from build123d import *

# Parameters (mm, degrees)
BOX013_W     = 26
BOX013_H     = 26
BOX013_DEPTH = 3
BOX014_W     = 5
BOX014_H     = 5
BOX014_DEPTH = 9
BOX012_W     = 30
BOX012_H     = 30
BOX012_DEPTH = 2
BOX015_W     = 5
BOX015_H     = 5
BOX015_DEPTH = 9
FILLET001_R  = 2
FILLET002_R  = 2


with BuildPart() as obj1:
    # Box013 → Box013 (new body)
    with BuildSketch(Plane(origin=(-13, -13, -10), x_dir=(1, 0, 0), z_dir=(0, 0, 1))):
        with Locations((13, 13)):
            Rectangle(BOX013_W, BOX013_H)
    extrude(amount=BOX013_DEPTH)


with BuildPart() as obj2:
    # Box014 → Box014 (new body)
    with BuildSketch(Plane(origin=(-13, 8, -7), x_dir=(1, 0, 0), z_dir=(0, 0, 1))):
        with Locations((2.5, 2.5)):
            Rectangle(BOX014_W, BOX014_H)
    extrude(amount=BOX014_DEPTH)


with BuildPart() as obj3:
    # Box012 → Box012 (new body)
    with BuildSketch(Plane(origin=(-15, -15, -12), x_dir=(1, 0, 0), z_dir=(0, 0, 1))):
        with Locations((15, 15)):
            Rectangle(BOX012_W, BOX012_H)
    extrude(amount=BOX012_DEPTH)


with BuildPart() as fillet002:
    # Box015 → Box015 (new body)
    with BuildSketch(Plane(origin=(8, -13, -7), x_dir=(1, 0, 0), z_dir=(0, 0, 1))):
        with Locations((2.5, 2.5)):
            Rectangle(BOX015_W, BOX015_H)
    extrude(amount=BOX015_DEPTH)

    # Fusion004: union obj1, obj2, obj3
    add(obj1.part)
    add(obj2.part)
    add(obj3.part)

    # Fillet001
    fillet001_edges = [fillet002.edges().sort_by_distance(p)[0] for p in [
        (-15, -15, -11),
        (-15, 15, -11),
        (15, 15, -11),
        (15, -15, -11),
    ]]
    fillet(fillet001_edges, radius=FILLET001_R)

    # Fillet002
    fillet002_edges = [fillet002.edges().sort_by_distance(p)[0] for p in [
        (-8, 8, -2.5),
        (8, -8, -2.5),
    ]]
    fillet(fillet002_edges, radius=FILLET002_R)


solid = fillet002.part
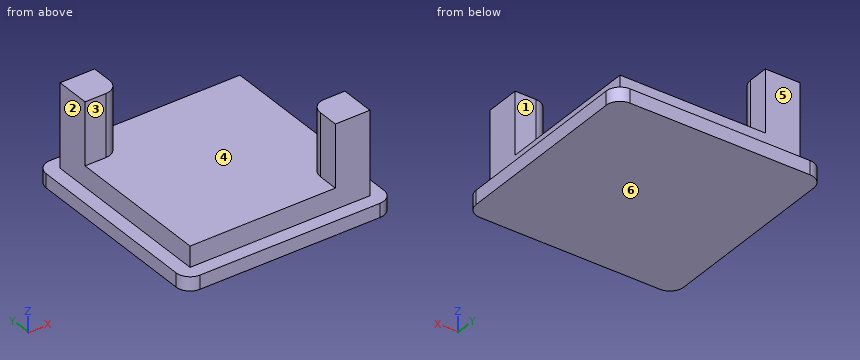
Check sheet for the modelled part. Datum: model origin and axes. Units: mm. Face numbers are marked on the shaded views. A direction names the side the tool comes from. Round coordinates to 2 decimals unless told otherwise and drop trailing zeros. Order: outer loops, then holes, each group sorted by start corner. A loop starts at its lowest first (then second) coordinate and runs counter-clockwise, first axis right, second up.
Q1. Set-up check for the marked faces 1, 2 and 3: record each of +Z, -Z, +X, -X, +Y, -Y from which the full face is reachable in a straight line by a thin tool's end or side.
Filled sheet:
face 1: +Z, +X, -X, +Y
face 2: +Z, -X, +Y, -Y
face 3: +Z, +X, -X, -Y
Q2. Scan lines: L1, parallel to Z at x = -11, y = 5.25; L2, parallel to X at y = 10, z = -2.25; L3, parallel to X at y = -10.5, z = -9.75. Record each from-to range of solid material in increasing order.
Filled sheet:
L1: z = -12 to -7
L2: x = -13 to -8
L3: x = -13 to 13
Q3. Cross-section at C-C, the plane y = -0.25. Enter the section's corners in (x, z).
Filled sheet:
outline: (-15, -12) - (15, -12) - (15, -10) - (13, -10) - (13, -7) - (-13, -7) - (-13, -10) - (-15, -10) - close
Q4. Draft check along Z on the marked faces 4, 5 and 6. Enter one of: pulls with the +Z half, pulls with the -Z half, needs draft (parallel to the pull), parting line crosses it, or undercut.
Filled sheet:
face 4: pulls with the +Z half
face 5: needs draft
face 6: pulls with the -Z half
Q5. Depth check by flat-ended pin: P1, Ø3.5, axis at y = -4, z = -3.5, coming from the -X side; P2, Ø2.5, axis at x = 11, z = -1.5, coming from the +Y side; P3, Ø1.5, axis at x = -11, z = -0.5, coming from the -Y side; P4, Ø5, axis at y = 11, z = -1, coming from the -X side. Enter the tip coordinate at first touch or a pass-through.
Filled sheet:
P1: passes through
P2: stops at y = -8
P3: stops at y = 8
P4: stops at x = -13
Q6. Cross-section at A-A, the plane z = -1.5. Enter the section's corners in (x, y), plus the area to 3 significant figures.
Filled sheet:
outline: (-13, 8) - (-10, 8) arc R2 ccw to (-8, 10) - (-8, 13) - (-13, 13) - close; (8, -13) - (13, -13) - (13, -8) - (10, -8) arc R2 ccw to (8, -10) - close
area: 48.3 mm2
Q7. Cross-section at B-B, the plane x = 12.5. Enter the section's corners in (y, z), plus the area to 3 significant figures.
Filled sheet:
outline: (-15, -12) - (15, -12) - (15, -10) - (13, -10) - (13, -7) - (-8, -7) - (-8, 2) - (-13, 2) - (-13, -10) - (-15, -10) - close
area: 183 mm2
